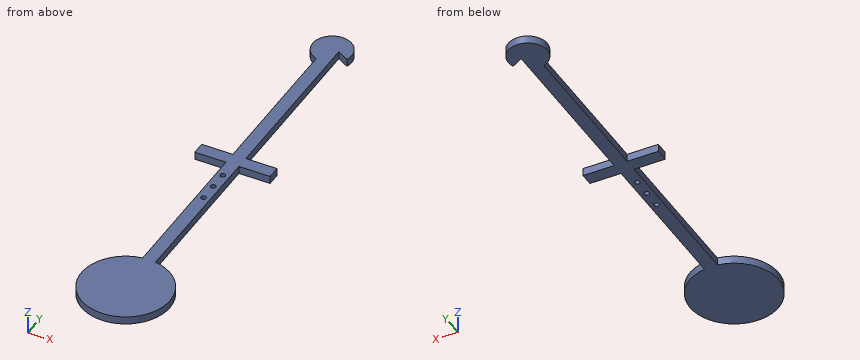
from build123d import *

# Parameters (mm, degrees)
F0_R     = 1
F1_DEPTH = 3


with BuildPart() as f1:
    # F0 (on Top) → F1 (new body)
    with BuildSketch(Plane.XY):
        with BuildLine():
            Line((-3.609526, 23.8211), (-3.609526, -36.712977))
            ThreePointArc((-3.609526, -36.712977), (-1.295909, -70.541409), (1.390474, -36.740537))
            Line((1.390474, -36.740537), (1.390474, 23.8211))
            Line((1.390474, 23.8211), (13.390474, 23.8211))
            Line((13.390474, 23.8211), (13.390474, 28.8211))
            Line((13.390474, 28.8211), (1.390474, 28.8211))
            Line((1.390474, 28.8211), (1.390474, 89.420719))
            Line((1.390474, 89.420719), (1.390474, 96.458332))
            Line((1.390474, 96.458332), (5.837989, 93.872674))
            ThreePointArc((5.837989, 93.872674), (-4.437612, 103.224584), (-3.609526, 89.355177))
            Line((-3.609526, 89.355177), (-3.609526, 28.8211))
            Line((-3.609526, 28.8211), (-15.609526, 28.8211))
            Line((-15.609526, 28.8211), (-15.609526, 23.8211))
            Line((-15.609526, 23.8211), (-3.609526, 23.8211))
        make_face()
        with Locations((-1.109526, 2.8211)):
            Circle(F0_R, mode=Mode.SUBTRACT)
        with Locations((-1.109526, 9.8211)):
            Circle(F0_R, mode=Mode.SUBTRACT)
        with Locations((-1.109526, 16.8211)):
            Circle(F0_R, mode=Mode.SUBTRACT)
    extrude(amount=F1_DEPTH)


solid = f1.part
Check sheet for the modelled part. Datum: model origin and axes. Units: mm. Give positions to 0.01 mm unless a question says otherwise; leave off trailing zeros. Loops run counter-clockwise (first coordinate to the right, second up) from the corner with the lowest first, then second, coordinate; pieces in that order, holes last. Notation, with made-up numbers: M 89,52.5 L 115,52.5 A12 ccw 115,67.5 Z; hole C 80,60 d8. An arc over 180 degrees is marked long. Answer as a JSON object with one key per item and string values. Group by question number.
Q1. Go/stop test with flat-tipped pins: P1, Ø1.5, axis at x = -12.5, z = 2, coming from the -Y side; P2, Ø0.9, axis at y = 59, z = 1.5, coming from the +X side; P3, Ø0.9, axis at y = 27.5, z = 1.5, coming from the +X side. Record where each tip stops, or that it passes through.
Q2. Cross-section at C-C on x = 3.5. Record the cut outline in (y, z).
Q3. Material ranges on line 1 along Y through (x, z) = (-6.5, 0.5); line 2 along X through (y, z) = (-4, 2); line 3 along Y through (x, z) = (-4.5, 1.1), recorded low to high. Write a range as [from, to].
Q4. Cross-section at D-D on y = 83. Record the cut outline in (x, z), then the cut area to 3 significant figures.
Q5. Cross-section at B-B on z = 1.1. Record the cut outline in (x, y).
Q6. Cross-section at A-A on x = -11. Record the cut outline in (y, z).
Evaluation:
{
 "1": {"P1": "stops at y = -66.87", "P2": "stops at x = 1.39", "P3": "stops at x = 13.39"},
 "2": {"outline": "M -69.88,0 L -37.2,0 L -37.2,3 L -69.88,3 Z; M 23.82,0 L 28.82,0 L 28.82,3 L 23.82,3 Z; M 95.23,0 L 102.3,0 L 102.3,3 L 95.23,3 Z"},
 "3": {"line 1": "y = [-69.7, -37.39], [23.82, 28.82], [91.15, 101.77]", "line 2": "x = [-3.61, 1.39]", "line 3": "y = [-70.22, -36.86], [23.82, 28.82], [89.72, 103.19]"},
 "4": {"outline": "M -3.61,0 L 1.39,0 L 1.39,3 L -3.61,3 Z", "area": "15.0 mm2"},
 "5": {"outline": "M -15.61,23.82 L -3.61,23.82 L -3.61,-36.71 A17 ccw long 1.39,-36.74 L 1.39,23.82 L 13.39,23.82 L 13.39,28.82 L 1.39,28.82 L 1.39,96.46 L 5.84,93.87 A7.5 ccw long -3.61,89.36 L -3.61,28.82 L -15.61,28.82 Z; hole C -1.11,2.82 d2; hole C -1.11,9.82 d2; hole C -1.11,16.82 d2"},
 "6": {"outline": "M -67.43,0 L -39.65,0 L -39.65,3 L -67.43,3 Z; M 23.82,0 L 28.82,0 L 28.82,3 L 23.82,3 Z"}
}
